CAD build for the part. Positions are in the model's coordinates, mm. A direction names the side the tool comes from. Coordinates: 2 decimals unless noted, no trailing zeros. Order: outer loops, then holes, each group sorted by start corner. A loop starts at its lowest first (then second) coordinate and runs counter-clockwise, first axis right, second up. Notation, with made-up numbers: (-8.75, -6.75) - (11.25, -6.75) arc R9 ccw to (11.25, 5.25) - close; hole circle Ø2 at (82, 61). An arc over 180 degrees is marked (long way). Use one line per item in the form item = value.
```python
from build123d import *

# Parameters (mm, degrees)
SKETCH_1_W      = 56
SKETCH_1_H      = 48.5
SKETCH_1_R      = 1
EXTRUDE_1_DEPTH = 1.5
SKETCH_2_W      = 6
SKETCH_2_H      = 35
EXTRUDE_2_DEPTH = 2.5
SKETCH_3_W      = 6
SKETCH_3_H      = 12
EXTRUDE_3_DEPTH = 4.5


with BuildPart() as part:
    # Эскиз1 → Бобышка-Вытянуть1 (new body)
    with BuildSketch(Plane(origin=(0, 0, 0), x_dir=(1, 0, 0), z_dir=(0, 1, 0))):
        Rectangle(SKETCH_1_W, SKETCH_1_H)
        with Locations(Location((-13, 21.25, 0), (0, 0, 270))):
            Circle(SKETCH_1_R, mode=Mode.SUBTRACT)
        with Locations(Location((-4, 21.25, 0), (0, 0, 270))):
            Circle(SKETCH_1_R, mode=Mode.SUBTRACT)
    extrude(amount=EXTRUDE_1_DEPTH)

    # Эскиз2 → Бобышка-Вытянуть2 (add)
    with BuildSketch(Plane(origin=(0, 1.5, 0), x_dir=(1, 0, 0), z_dir=(0, 1, 0))):
        with Locations((3.5, -0.75)):
            Rectangle(SKETCH_2_W, SKETCH_2_H)
        with Locations((13.5, -0.75)):
            Rectangle(SKETCH_2_W, SKETCH_2_H)
    extrude(amount=EXTRUDE_2_DEPTH)

    # Эскиз3 → Бобышка-Вытянуть3 (add)
    with BuildSketch(Plane.XZ):
        with Locations((-25.5, -7.25)):
            Rectangle(SKETCH_3_W, SKETCH_3_H)
    extrude(amount=EXTRUDE_3_DEPTH)


solid = part.part
```
Item 1: Cut at B-B, the plane x = -13. Write the cut outline in (y, z).
Derived:
outline = (0, -24.25) - (1.5, -24.25) - (1.5, -22.25) - (0, -22.25) - close; (0, -20.25) - (1.5, -20.25) - (1.5, 24.25) - (0, 24.25) - close
Item 2: Cut at C-C, the plane z = -10. Write the cut outline in (x, y), plus the area to 3 significant figures.
Derived:
outline = (-28.5, -4.5) - (-22.5, -4.5) - (-22.5, 0) - (28, 0) - (28, 1.5) - (16.5, 1.5) - (16.5, 4) - (10.5, 4) - (10.5, 1.5) - (6.5, 1.5) - (6.5, 4) - (0.5, 4) - (0.5, 1.5) - (-28, 1.5) - (-28, 0) - (-28.5, 0) - close
area = 141 mm²
Item 3: 3-axis set-ups, long thin cutter, end or side, ignore diameter. For faces 4 (the face through (-28, 1, 0)), 5 (the face through (3, 3, 18.25)), 6 (the face through (-26, -2, -1.25)), 7 (the face through (16.5, 3, 1)): which of +Z, -Z, +X, -X, +Y, -Y reach the whole face in a straight line?
Derived:
face_4 = +Z, -Z, -X, +Y
face_5 = +Z, +X, -X, +Y
face_6 = +Z, +X, -X, -Y
face_7 = +Z, -Z, +X, +Y
Item 4: Two-plate mould, pull along X, no slides. Class faces 1 (the face through (13, 3, -16.75)), 2 (the face through (-3.324, 0.74, -21.987)), 3 (the face through (-22.5, -2, -7)): +X half, -X half, draft (parallel to the pull), parting line (faces both ways), or undercut.
Derived:
face_1 = draft
face_2 = undercut
face_3 = +X half
Item 5: Drill centre lines: line 1 (X direction, y = 0.45, z = -21.25); line 2 (X direction, y = 3.25, z = -8); line 3 (Y direction, x = 1.5, z = 13.5). Where is each one in solid material? Low to high. Write a range as [from, to].
Derived:
line_1 = [-28, -14], [-12, -5], [-3, 28]
line_2 = [0.5, 6.5], [10.5, 16.5]
line_3 = [0, 4]
Item 6: Cut at A-A, the plane z = -21.25. Write the cut outline in (x, y), plus the area to 3 significant figures.
Derived:
outline = (-28, 0) - (-14, 0) - (-14, 1.5) - (-28, 1.5) - close; (-12, 0) - (-5, 0) - (-5, 1.5) - (-12, 1.5) - close; (-3, 0) - (28, 0) - (28, 1.5) - (-3, 1.5) - close
area = 78.0 mm²
Item 7: Cut at D-D, the plane x = 13.5. Write the cut outline in (y, z).
Derived:
outline = (0, -24.25) - (1.5, -24.25) - (1.5, -16.75) - (4, -16.75) - (4, 18.25) - (1.5, 18.25) - (1.5, 24.25) - (0, 24.25) - close
Item 8: Drop flat-ended pins along their axis: pin 1 (3 mm diameter, centred on x = -4, z = -21.25, fed in from -Y); pin 2 (0.8 mm diameter, centred on x = 3, y = 3.5, fed in from +Z); pin 3 (5 mm diameter, centred on x = -24.5, y = -3.5, fed in from -Z). Give the stop position or say it passes through.
Derived:
pin_1 = 0
pin_2 = 18.25
pin_3 = -13.25
